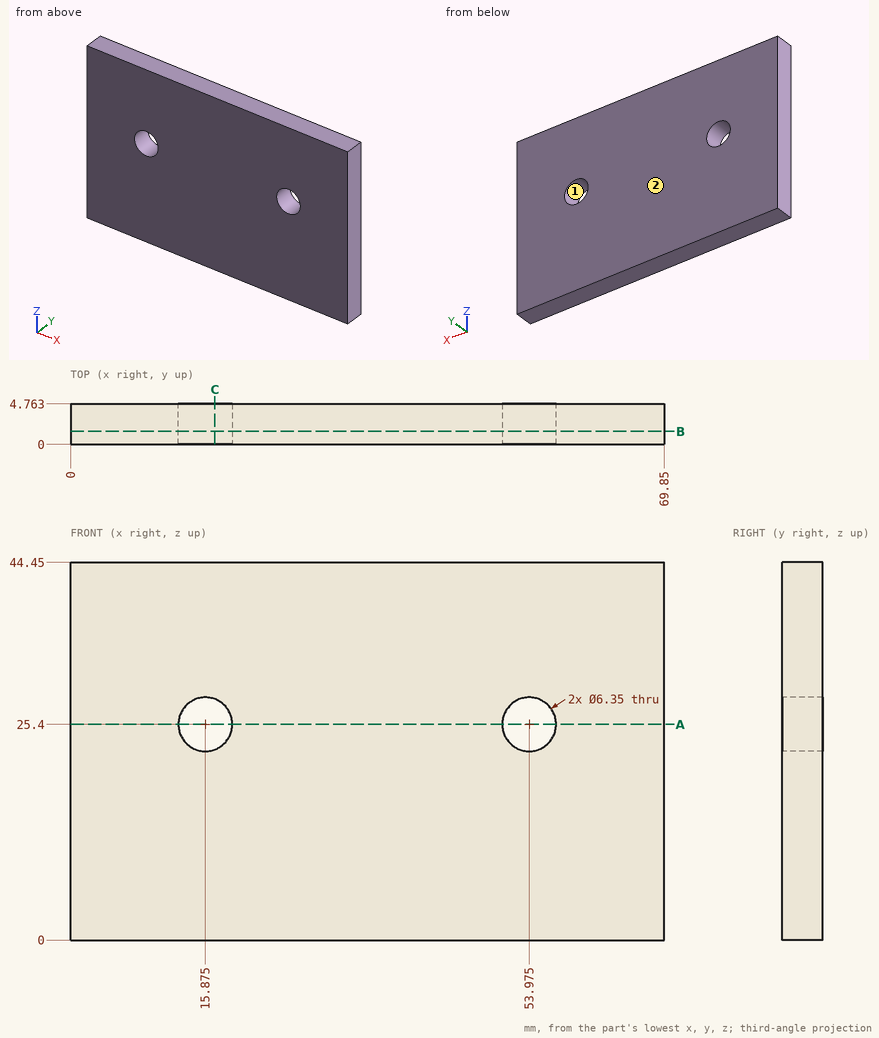
Geometry check sheet. Reference: drawing and pictorial views, mm from the part's lowest x, y, z. Coordinates: 2 decimals unless noted, no trailing zeros. Write each loop counter-clockwise with the first axis right and the second up, starting at its lowest first coordinate (ties: lowest second). Pieces come first, ordered by that corner, then holes. Notation, with made-up numbers: M 30,-33 L 76,-33 A17 cw 76,-29 Z; hole C -5,53 d8. An arc over 180 degrees is marked long. Use one line per item in the form item = value.
Item 1: Release check for a two-part mould opening along Z. For the marked faces 1 and 2 record: pulls with the +Z half, pulls with the -Z half, needs draft (parallel to the pull), parting line crosses it, or undercut.
Answer below:
face_1 = undercut
face_2 = needs draft
Item 2: Sectioned sample at B-B, the plane y = 1.55. State how many separate pieces and enclosed holes the cut face has, and give its area (3 significant figures).
Answer below:
separate_pieces = 1
enclosed_holes = 2
area = 3,040 mm^2
Item 3: Material ranges on L1, parallel to Z at x = 51.5, y = 3.15, recorded low to high. Write a range as from..to.
Answer below:
L1 = 0..23.41, 27.39..44.45
Item 4: Sectioned sample at C-C, the plane x = 17. Record the cut outline in (y, z).
Answer below:
outline = M 0,0 L 4.76,0 L 4.76,22.43 L 0,22.43 Z; M 0,28.37 L 4.76,28.37 L 4.76,44.45 L 0,44.45 Z
Item 5: Sectioned sample at A-A, the plane z = 25.4. Record the cut outline in (x, y), and give its area (3 significant figures).
Answer below:
outline = M 0,0 L 12.7,0 L 12.7,4.76 L 0,4.76 Z; M 19.05,0 L 50.8,0 L 50.8,4.76 L 19.05,4.76 Z; M 57.15,0 L 69.85,0 L 69.85,4.76 L 57.15,4.76 Z
area = 272 mm^2
